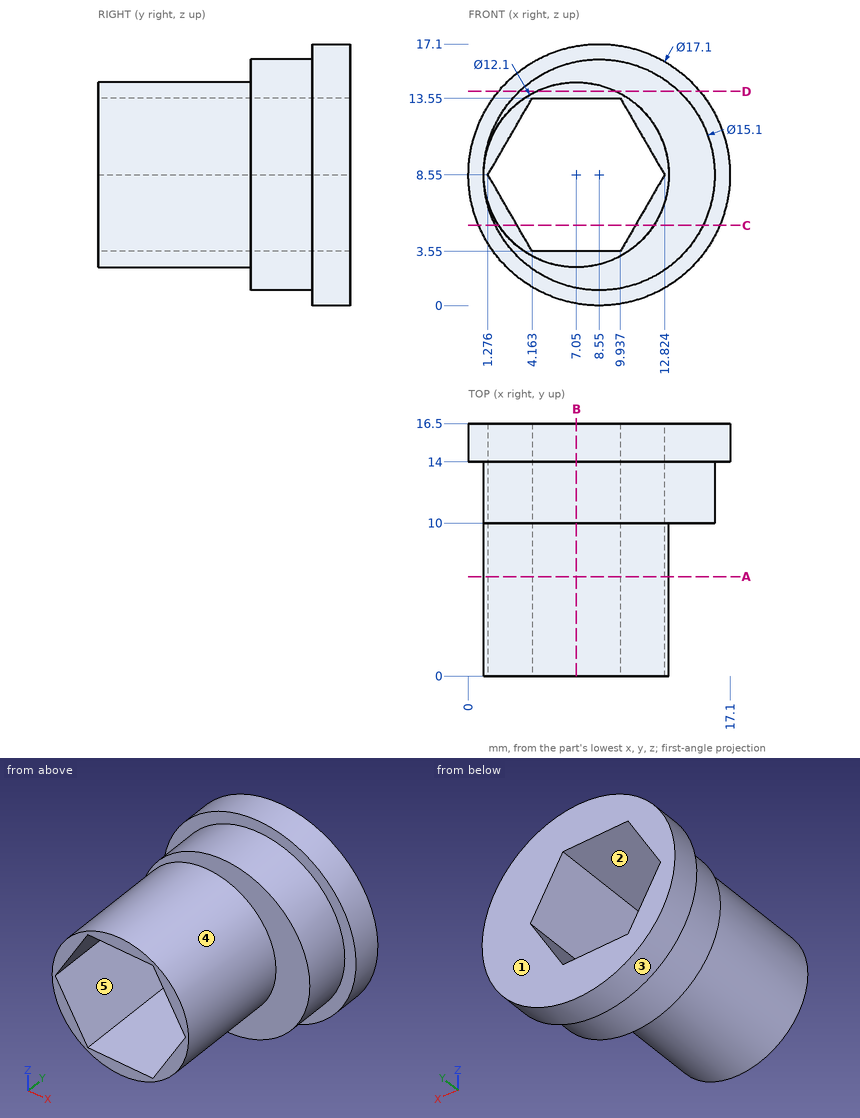
Design review of the part shown in the three views and the two pictorial views. Dimensions are in mm from the part's minimum x, y and z. A direction names the side the tool comes from. Coordinates: 2 decimals unless noted, no trailing zeros. Write each loop counter-clockwise with the first axis right and the second up, starting at its lowest first coordinate (ties: lowest second). Pieces come first, ordered by that corner, then holes.
(1) Add section B-B on x = 7.05. Give the boundary of the cut face in (y, z).
(2) For pin 1 Ø4.5 at (x, y) = (8.5, 8) entering from -Z; pin 2 Ø1.7 at (x, y) = (6.5, 6) entering from +Z; pin 3 Ø3 at (x, y) = (12.5, 10) entering from +Z, all flat-tipped, find the tip position at first contact; note any pin that passes through.
(3) Wall thickness on probe 1 along Y at (x, z) = (11.5, 2.25); probe 2 along X at (y, z) = (12, 6.75) (1 decimal); probe 3 along X at (y, z) = (5, 8.5) (1 decimal): over which ranges is each line inside the solid? List them lowest first.
(4) Add section D-D on z = 14. Give the boundary of the cut face in (x, y) (1 decimal), then the cut area to 3 significant figures.
(5) Tool access review of the marked faces 4 and 5: name each direction out of +Z, -Z, +X, -X, +Y, -Y from which nothing blocks a thin tool from reaching the whole face with its end or side.
(6) Add section C-C on z = 5.25. Give the boundary of the cut face in (x, y).
(7) Add section A-A on y = 6.5. Give the boundary of the cut face in (x, z).
(8) The part is to be moulded in two halves that separate along Z. For the marked faces 1, 2 and 3, say which applies: +Z half, -Z half, draft (parallel to the pull), parting line (faces both ways), or undercut.
Answer sheet:
1. outline: (0, 2.5) - (10, 2.5) - (10, 1.15) - (14, 1.15) - (14, 0.13) - (16.5, 0.13) - (16.5, 3.55) - (0, 3.55) - close; (0, 13.55) - (16.5, 13.55) - (16.5, 16.97) - (14, 16.97) - (14, 15.95) - (10, 15.95) - (10, 14.6) - (0, 14.6) - close
2. pin 1: stops at z = 1
2. pin 2: stops at z = 14.6
2. pin 3: stops at z = 15.69
3. probe 1: y = 10 to 16.5
3. probe 2: x = 1.2 to 2.3, 11.8 to 15.9
3. probe 3: x = 1 to 1.3, 12.8 to 13.1
4. outline: (2, 14) - (3.3, 14) - (3.3, 10) - (4.4, 10) - (4.4, 0) - (9.7, 0) - (9.7, 10) - (13.8, 10) - (13.8, 14) - (15.1, 14) - (15.1, 16.5) - (2, 16.5) - close
4. area: 127 mm2
5. face 4: -Y
5. face 5: +Y, -Y
6. outline: (0.66, 14) - (1.76, 14) - (1.76, 10) - (1.98, 10) - (1.98, 0) - (3.18, 0) - (3.18, 16.5) - (0.66, 16.5) - close; (10.92, 0) - (12.12, 0) - (12.12, 10) - (15.34, 10) - (15.34, 14) - (16.44, 14) - (16.44, 16.5) - (10.92, 16.5) - close
7. outline: circle Ø12.1 at (7.05, 8.55); hole (1.28, 8.55) - (4.16, 3.55) - (9.94, 3.55) - (12.82, 8.55) - (9.94, 13.55) - (4.16, 13.55) - close
8. face 1: draft
8. face 2: undercut
8. face 3: parting line
